from build123d import *

# Parameters (mm, degrees)
SKETCH1_W           = 64.516
SKETCH1_H           = 119.888
BOSS_EXTRUDE1_DEPTH = 13.081
SKETCH2_W           = 58.42
SKETCH2_H           = 113.792
CUT_EXTRUDE1_DEPTH  = 10.16
SKETCH3_W           = 56.896
SKETCH3_H           = 3.048
BOSS_EXTRUDE2_DEPTH = 23.2156
SKETCH4_R           = 2.9591
SKETCH4_R_2         = 1.1684
BOSS_EXTRUDE3_DEPTH = 4.826
SKETCH5_R           = 5.0165
CUT_EXTRUDE2_DEPTH  = 141.176237199
SKETCH6_R           = 3.175
SKETCH6_R_2         = 2.159
BOSS_EXTRUDE4_DEPTH = 8.763
SKETCH6_2_R         = 2.159
CUT_EXTRUDE3_DEPTH  = 141.176237199


with BuildPart() as part:
    # Sketch1 → Boss-Extrude1 (new body)
    with BuildSketch(Plane(origin=(0, 0, 0), x_dir=(1, 0, 0), z_dir=(0, 1, 0))):
        with Locations((32.258, 59.944)):
            Rectangle(SKETCH1_W, SKETCH1_H)
    extrude(amount=BOSS_EXTRUDE1_DEPTH)

    # Sketch2 → Cut-Extrude1 (cut)
    with BuildSketch(Plane(origin=(0, 13.081, 0), x_dir=(1, 0, 0), z_dir=(0, 1, 0))):
        with Locations((32.258, 59.944)):
            Rectangle(SKETCH2_W, SKETCH2_H)
    extrude(amount=-CUT_EXTRUDE1_DEPTH, mode=Mode.SUBTRACT)

    # Sketch3 → Boss-Extrude2 (add)
    with BuildSketch(Plane(origin=(0, 13.081, 0), x_dir=(1, 0, 0), z_dir=(0, 1, 0))):
        with Locations((32.258, 1.524)):
            Rectangle(SKETCH3_W, SKETCH3_H)
        with Locations((32.258, 118.364)):
            Rectangle(SKETCH3_W, SKETCH3_H)
    extrude(amount=BOSS_EXTRUDE2_DEPTH)

    # Sketch4 → Boss-Extrude3 (add)
    # profile 1 of 6: a face of its own
    with BuildSketch(Plane(origin=(0, 2.921, 0), x_dir=(1, 0, 0), z_dir=(0, 1, 0))):
        with Locations(Location((8.3566, 102.87, 0), (0, 0, 270))):
            Circle(SKETCH4_R)
        with Locations(Location((8.3566, 102.87, 0), (0, 0, 270))):
            Circle(SKETCH4_R_2, mode=Mode.SUBTRACT)
    # profile 2 of 6: a face of its own
    with BuildSketch(Plane(origin=(0, 2.921, 0), x_dir=(1, 0, 0), z_dir=(0, 1, 0))):
        with Locations(Location((56.1594, 102.87, 0), (0, 0, 270))):
            Circle(SKETCH4_R)
        with Locations(Location((56.1594, 102.87, 0), (0, 0, 270))):
            Circle(SKETCH4_R_2, mode=Mode.SUBTRACT)
    # profile 3 of 6: a face of its own
    with BuildSketch(Plane(origin=(0, 2.921, 0), x_dir=(1, 0, 0), z_dir=(0, 1, 0))):
        with Locations(Location((10.7442, 72.0852, 0), (0, 0, 270))):
            Circle(SKETCH4_R)
        with Locations(Location((10.7442, 72.0852, 0), (0, 0, 270))):
            Circle(SKETCH4_R_2, mode=Mode.SUBTRACT)
    # profile 4 of 6: a face of its own
    with BuildSketch(Plane(origin=(0, 2.921, 0), x_dir=(1, 0, 0), z_dir=(0, 1, 0))):
        with Locations(Location((53.7718, 72.0852, 0), (0, 0, 270))):
            Circle(SKETCH4_R)
        with Locations(Location((53.7718, 72.0852, 0), (0, 0, 270))):
            Circle(SKETCH4_R_2, mode=Mode.SUBTRACT)
    # profile 5 of 6: a face of its own
    with BuildSketch(Plane(origin=(0, 2.921, 0), x_dir=(1, 0, 0), z_dir=(0, 1, 0))):
        with Locations(Location((10.7442, 17.018, 0), (0, 0, 270))):
            Circle(SKETCH4_R)
        with Locations(Location((10.7442, 17.018, 0), (0, 0, 270))):
            Circle(SKETCH4_R_2, mode=Mode.SUBTRACT)
    # profile 6 of 6: a face of its own
    with BuildSketch(Plane(origin=(0, 2.921, 0), x_dir=(1, 0, 0), z_dir=(0, 1, 0))):
        with Locations(Location((53.7718, 17.018, 0), (0, 0, 270))):
            Circle(SKETCH4_R)
        with Locations(Location((53.7718, 17.018, 0), (0, 0, 270))):
            Circle(SKETCH4_R_2, mode=Mode.SUBTRACT)
    extrude(amount=BOSS_EXTRUDE3_DEPTH)

    # Sketch5 → Cut-Extrude2 (cut, through all)
    with BuildSketch(Plane(origin=(0, 2.921, 0), x_dir=(1, 0, 0), z_dir=(0, 1, 0))):
        with Locations(Location((31.1785, 82.8675, 0), (0, 0, 270))):
            Circle(SKETCH5_R)
    extrude(amount=-CUT_EXTRUDE2_DEPTH, mode=Mode.SUBTRACT)

    # Sketch6 → Boss-Extrude4 (add)
    # profile 1 of 4: a face of its own
    with BuildSketch(Plane(origin=(0, 2.921, 0), x_dir=(1, 0, 0), z_dir=(0, 1, 0))):
        with Locations(Location((8.3058, 111.3155, 0), (0, 0, 270))):
            Circle(SKETCH6_R)
        with Locations(Location((8.3058, 111.3155, 0), (0, 0, 270))):
            Circle(SKETCH6_R_2, mode=Mode.SUBTRACT)
    # profile 2 of 4: a face of its own
    with BuildSketch(Plane(origin=(0, 2.921, 0), x_dir=(1, 0, 0), z_dir=(0, 1, 0))):
        with Locations(Location((56.2102, 111.3155, 0), (0, 0, 270))):
            Circle(SKETCH6_R)
        with Locations(Location((56.2102, 111.3155, 0), (0, 0, 270))):
            Circle(SKETCH6_R_2, mode=Mode.SUBTRACT)
    # profile 3 of 4: a face of its own
    with BuildSketch(Plane(origin=(0, 2.921, 0), x_dir=(1, 0, 0), z_dir=(0, 1, 0))):
        with Locations(Location((8.3058, 8.5725, 0), (0, 0, 270))):
            Circle(SKETCH6_R)
        with Locations(Location((8.3058, 8.5725, 0), (0, 0, 270))):
            Circle(SKETCH6_R_2, mode=Mode.SUBTRACT)
    # profile 4 of 4: a face of its own
    with BuildSketch(Plane(origin=(0, 2.921, 0), x_dir=(1, 0, 0), z_dir=(0, 1, 0))):
        with Locations(Location((56.2102, 8.5725, 0), (0, 0, 270))):
            Circle(SKETCH6_R)
        with Locations(Location((56.2102, 8.5725, 0), (0, 0, 270))):
            Circle(SKETCH6_R_2, mode=Mode.SUBTRACT)
    extrude(amount=BOSS_EXTRUDE4_DEPTH)

    # Sketch6_2 → Cut-Extrude3 (cut, through all)
    with BuildSketch(Plane(origin=(0, 2.921, 0), x_dir=(1, 0, 0), z_dir=(0, 1, 0))):
        with Locations(Location((8.3058, 111.3155, 0), (0, 0, 270))):
            Circle(SKETCH6_2_R)
        with Locations(Location((56.2102, 111.3155, 0), (0, 0, 270))):
            Circle(SKETCH6_2_R)
        with Locations(Location((8.3058, 8.5725, 0), (0, 0, 270))):
            Circle(SKETCH6_2_R)
        with Locations(Location((56.2102, 8.5725, 0), (0, 0, 270))):
            Circle(SKETCH6_2_R)
    extrude(amount=-CUT_EXTRUDE3_DEPTH, mode=Mode.SUBTRACT)


solid = part.part
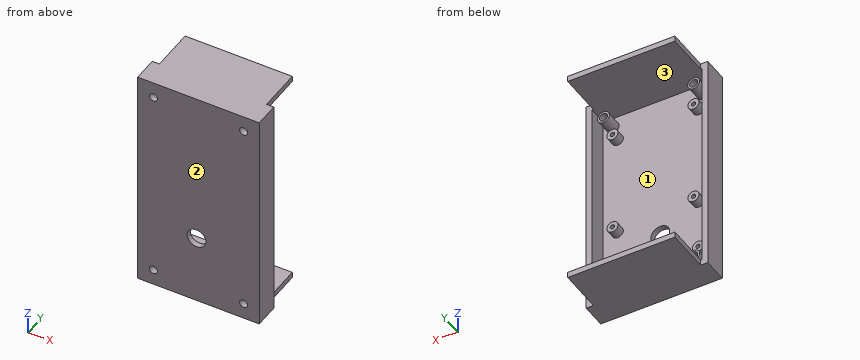
The listing builds one solid part. Answer for the finished solid, in the listing's coordinates (mm). Face numbers are marked on the shaded views. Give positions to 0.01 mm unless a question says otherwise; leave off trailing zeros. Write each loop counter-clockwise with the first axis right and the second up, starting at its lowest first coordinate (ties: lowest second). Pieces come first, ordered by that corner, then holes. Notation, with made-up numbers: (21, 28.5) -> (37, 28.5) arc R34 cw to (37, 61.5) -> close; hole circle Ø2 at (27.25, 75.25). An arc over 180 degrees is marked (long way). One line per question, with ' | ' between items. Start each with the question number.
1. Section B-B (z = -92) is taken. Determine the outline of the cut face in (x, y).
2. Section A-A (y = 18) is taken. Determine the outline of the cut face in (x, z).
3. For a pull along X with two mould halves and no side action, classify the marked faces 1, 2 and 3 as pulls with the +X half, pulls with the -X half, needs draft (parallel to the pull), parting line crosses it, or undercut.
4. Find the intervals of material crossed by probe 1 along X at (y, z) = (5, -102.87) (1 decimal); probe 2 along Z at (x, y) = (31, 16); probe 3 along X at (y, z) = (6, -102), in increasing order.
5. Section C-C (x = 20) is taken. Determine the outline of the cut face in (y, z).
6. Given pin 1 Ø5 at (x, z) = (56.21, -8.57) entering from +Y; pin 2 Ø16 at (x, z) = (31.18, -82.87) entering from +Y; pin 3 Ø2.5 at (y, z) = (22.5, -2) entering from -X, each flat-ended and moving along its own axis, determine where each tip first touches the part or whether it passes through.
Response values:
1) outline: (0, 0) -> (64.52, 0) -> (64.52, 13.08) -> (61.47, 13.08) -> (61.47, 2.92) -> (3.05, 2.92) -> (3.05, 13.08) -> (0, 13.08) -> close
2) outline: (3.81, -119.89) -> (60.71, -119.89) -> (60.71, -116.84) -> (3.81, -116.84) -> close; (3.81, -3.05) -> (60.71, -3.05) -> (60.71, 0) -> (3.81, 0) -> close
3) face 1: undercut | face 2: needs draft | face 3: undercut
4) probe 1: 0 to 3, 5.4 to 7.2, 9.5 to 11.3, 53.2 to 55, 57.3 to 59.1, 61.5 to 64.5 | probe 2: -119.89 to -116.84, -3.05 to 0 | probe 3: 0 to 3.05, 5.53 to 7.58, 9.14 to 11.18, 53.33 to 55.38, 56.94 to 58.99, 61.47 to 64.52
5) outline: (0, -119.89) -> (36.3, -119.89) -> (36.3, -116.84) -> (2.92, -116.84) -> (2.92, -3.05) -> (36.3, -3.05) -> (36.3, 0) -> (0, 0) -> close
6) pin 1: y = 11.68 | pin 2: y = 2.92 | pin 3: x = 3.81
